from build123d import *

# Parameters (mm, degrees)
SKETCH_23_R                      = 1.6
SKETCH_23_R_2                    = 2.15
EXTRUDE_9_DEPTH                  = 12
SKETCH_25_R                      = 3.199536645
SKETCH_25_R_2                    = 3.253572192
SKETCH_25_R_3                    = 3.504037636
EXTRUDE_11_DEPTH                 = 8.5
SKETCH_27_R                      = 2.9
CUT_EXTRUDE_14_DEPTH             = 15
CUT_EXTRUDE_14_DEPTH_BACK        = 5
EXTRUDE_14_DEPTH                 = 48
EXTRUDE_14_DEPTH_BACK            = 8.5
EXTRUDE_15_REACH                 = 62
SKETCH_30_R                      = 2.823102459
SKETCH_30_R_2                    = 3.099807243
CUT_EXTRUDE_15_DEPTH             = 38
CUT_EXTRUDE_16_REACH             = 8
SKETCH_33_R                      = 1.4
CUT_EXTRUDE_16_DIRECTION_2_REACH = 56


with BuildPart() as part:
    # 草图23 → 凸台-拉伸9 (new body)
    with BuildSketch(Plane(origin=(10, 0, 0), x_dir=(0, 0, -1), z_dir=(1, 0, 0))):
        with BuildLine():
            Line((32.5, 0), (32.5, 29))
            Line((32.5, 29), (27, 29))
            Line((27, 29), (27, 13.076696831))
            ThreePointArc((27, 13.076696831), (-30, 0), (27, -13.076696831))
            Line((27, -13.076696831), (27, -29))
            Line((27, -29), (32.5, -29))
            Line((32.5, -29), (32.5, 0))
        make_face()
        with Locations((0, 12.5)):
            Circle(SKETCH_23_R, mode=Mode.SUBTRACT)
        with Locations((-10.825317547, 6.25)):
            Circle(SKETCH_23_R, mode=Mode.SUBTRACT)
        with Locations((10.825317547, 6.25)):
            Circle(SKETCH_23_R, mode=Mode.SUBTRACT)
        with Locations((10.825317547, -6.25)):
            Circle(SKETCH_23_R, mode=Mode.SUBTRACT)
        with Locations((0, -12.5)):
            Circle(SKETCH_23_R, mode=Mode.SUBTRACT)
        with Locations((-10.825317547, -6.25)):
            Circle(SKETCH_23_R, mode=Mode.SUBTRACT)
        with Locations((5.1, 8.833459119)):
            Circle(SKETCH_23_R_2, mode=Mode.SUBTRACT)
        with Locations((-10.2, 0)):
            Circle(SKETCH_23_R_2, mode=Mode.SUBTRACT)
        with Locations((5.1, -8.833459119)):
            Circle(SKETCH_23_R_2, mode=Mode.SUBTRACT)
    extrude(amount=-EXTRUDE_9_DEPTH)

    # 草图25 → 凸台-拉伸11 (add)
    with BuildSketch(Plane(origin=(10, 0, 0), x_dir=(0, 0, -1), z_dir=(1, 0, 0))):
        with Locations((5.1, 8.833459119)):
            Circle(SKETCH_25_R)
        with Locations((-10.2, 0)):
            Circle(SKETCH_25_R_2)
        with Locations((5.1, -8.833459119)):
            Circle(SKETCH_25_R_3)
    extrude(amount=-EXTRUDE_11_DEPTH)

    # 草图27 → 切除-拉伸14 (cut, two sides)
    with BuildSketch(Plane(origin=(10, 0, 0), x_dir=(0, 0, -1), z_dir=(1, 0, 0))) as cut_extrude_14_sk:
        with Locations((0, 12.5)):
            Circle(SKETCH_27_R)
        with Locations((-86.65969357, 123.729949726)):
            Circle(SKETCH_27_R)
        with Locations((-33.661578231, 254.394420705)):
            Circle(SKETCH_27_R)
        with Locations((105.996230679, 273.828941958)):
            Circle(SKETCH_27_R)
        with Locations((192.655924249, 162.598992232)):
            Circle(SKETCH_27_R)
        with Locations((139.657808909, 31.934521253)):
            Circle(SKETCH_27_R)
        with Locations((10.825317547, 6.25)):
            Circle(SKETCH_27_R)
        with Locations((10.825317547, -6.25)):
            Circle(SKETCH_27_R)
        with Locations((0, -12.5)):
            Circle(SKETCH_27_R)
        with Locations((-10.825317547, -6.25)):
            Circle(SKETCH_27_R)
        with Locations((-10.825317547, 6.25)):
            Circle(SKETCH_27_R)
    extrude(amount=CUT_EXTRUDE_14_DEPTH, mode=Mode.SUBTRACT)
    extrude(cut_extrude_14_sk.sketch, amount=-CUT_EXTRUDE_14_DEPTH_BACK, mode=Mode.SUBTRACT)

    # 草图29 → 凸台-拉伸14 (add, two sides)
    with BuildSketch(Plane(origin=(10, 0, 0), x_dir=(0, 0, -1), z_dir=(1, 0, 0))) as extrude_14_sk:
        with BuildLine():
            Line((-7, 29.171904292), (-7, -29.171904292))
            ThreePointArc((-7, -29.171904292), (0, -30), (7, -29.171904292))
            Line((7, -29.171904292), (7, 29.171904292))
            ThreePointArc((7, 29.171904292), (0, 30), (-7, 29.171904292))
        make_face()
    extrude(amount=EXTRUDE_14_DEPTH)
    extrude(extrude_14_sk.sketch, amount=-EXTRUDE_14_DEPTH_BACK)

    # 草图30 → 凸台-拉伸15 (add, up to next)
    with BuildSketch(Plane.ZY.offset(2), mode=Mode.PRIVATE) as extrude_15_sk1:
        with Locations((0, 12.5)):
            Circle(SKETCH_30_R)
    extrude_15_tool1 = extrude(extrude_15_sk1.sketch, amount=-EXTRUDE_15_REACH, mode=Mode.PRIVATE) - part.part
    add(extrude_15_tool1.solids().sort_by_distance((-2, 12.5, 0))[0])
    # 草图30 → 凸台-拉伸15 (add, up to next)
    with BuildSketch(Plane.ZY.offset(2), mode=Mode.PRIVATE) as extrude_15_sk2:
        with Locations((0, -12.5)):
            Circle(SKETCH_30_R_2)
    extrude_15_tool2 = extrude(extrude_15_sk2.sketch, amount=-EXTRUDE_15_REACH, mode=Mode.PRIVATE) - part.part
    add(extrude_15_tool2.solids().sort_by_distance((-2, -12.5, 0))[0])

    # 草图32 → 切除-拉伸15 (cut, through all)
    with BuildSketch(Plane(origin=(0, 0, -7), x_dir=(-1, 0, 0), z_dir=(0, 0, -1))):
        Polygon((-58, 0), (-58, 24), (-10, 24), (-10, -24), (-58, -24), align=None)
    extrude(amount=-CUT_EXTRUDE_15_DEPTH, mode=Mode.SUBTRACT)

    # 草图33 → 切除-拉伸16 (cut, up to next)
    with BuildSketch(Plane(origin=(0, -24, 0), x_dir=(1, 0, 0), z_dir=(0, 1, 0)), mode=Mode.PRIVATE) as cut_extrude_16_sk1:
        with Locations((34.5, 0)):
            Circle(SKETCH_33_R)
    cut_extrude_16_tool1 = extrude(cut_extrude_16_sk1.sketch, amount=-CUT_EXTRUDE_16_REACH, mode=Mode.PRIVATE) & part.part
    add(cut_extrude_16_tool1.solids().sort_by_distance((34.5, -24, 0))[0], mode=Mode.SUBTRACT)
    # 草图33 → 切除-拉伸16 (cut, up to next)
    with BuildSketch(Plane(origin=(0, -24, 0), x_dir=(1, 0, 0), z_dir=(0, 1, 0)), mode=Mode.PRIVATE) as cut_extrude_16_sk2:
        with Locations((42, 0)):
            Circle(SKETCH_33_R)
    cut_extrude_16_tool2 = extrude(cut_extrude_16_sk2.sketch, amount=-CUT_EXTRUDE_16_REACH, mode=Mode.PRIVATE) & part.part
    add(cut_extrude_16_tool2.solids().sort_by_distance((42, -24, 0))[0], mode=Mode.SUBTRACT)
    # 草图33 → 切除-拉伸16 (cut, up to next)
    with BuildSketch(Plane(origin=(0, -24, 0), x_dir=(1, 0, 0), z_dir=(0, 1, 0)), mode=Mode.PRIVATE) as cut_extrude_16_sk3:
        with Locations((27, 0)):
            Circle(SKETCH_33_R)
    cut_extrude_16_tool3 = extrude(cut_extrude_16_sk3.sketch, amount=-CUT_EXTRUDE_16_REACH, mode=Mode.PRIVATE) & part.part
    add(cut_extrude_16_tool3.solids().sort_by_distance((27, -24, 0))[0], mode=Mode.SUBTRACT)

    # 草图33 → 切除-拉伸16 direction 2 (cut, up to next)
    with BuildSketch(Plane(origin=(0, -24, 0), x_dir=(1, 0, 0), z_dir=(0, 1, 0)), mode=Mode.PRIVATE) as cut_extrude_16_direction_2_sk1:
        with Locations((34.5, 0)):
            Circle(SKETCH_33_R)
    cut_extrude_16_direction_2_tool1 = extrude(cut_extrude_16_direction_2_sk1.sketch, amount=CUT_EXTRUDE_16_DIRECTION_2_REACH, mode=Mode.PRIVATE) & part.part
    add(cut_extrude_16_direction_2_tool1.solids().sort_by_distance((34.5, -24, 0))[0], mode=Mode.SUBTRACT)
    # 草图33 → 切除-拉伸16 direction 2 (cut, up to next)
    with BuildSketch(Plane(origin=(0, -24, 0), x_dir=(1, 0, 0), z_dir=(0, 1, 0)), mode=Mode.PRIVATE) as cut_extrude_16_direction_2_sk2:
        with Locations((42, 0)):
            Circle(SKETCH_33_R)
    cut_extrude_16_direction_2_tool2 = extrude(cut_extrude_16_direction_2_sk2.sketch, amount=CUT_EXTRUDE_16_DIRECTION_2_REACH, mode=Mode.PRIVATE) & part.part
    add(cut_extrude_16_direction_2_tool2.solids().sort_by_distance((42, -24, 0))[0], mode=Mode.SUBTRACT)
    # 草图33 → 切除-拉伸16 direction 2 (cut, up to next)
    with BuildSketch(Plane(origin=(0, -24, 0), x_dir=(1, 0, 0), z_dir=(0, 1, 0)), mode=Mode.PRIVATE) as cut_extrude_16_direction_2_sk3:
        with Locations((27, 0)):
            Circle(SKETCH_33_R)
    cut_extrude_16_direction_2_tool3 = extrude(cut_extrude_16_direction_2_sk3.sketch, amount=CUT_EXTRUDE_16_DIRECTION_2_REACH, mode=Mode.PRIVATE) & part.part
    add(cut_extrude_16_direction_2_tool3.solids().sort_by_distance((27, -24, 0))[0], mode=Mode.SUBTRACT)


solid = part.part
The listing builds one solid part. Answer for the finished solid, in the listing's coordinates (mm). A direction names the side the tool comes from. Round coordinates to 2 decimals unless told otherwise and drop trailing zeros. Write each loop counter-clockwise with the first axis right and the second up, starting at its lowest first coordinate (ties: lowest second). Pieces come first, ordered by that corner, then holes. Notation, with made-up numbers: (-7, 60.25) - (23, 60.25) arc R21 cw to (23, 75.25) - close; hole circle Ø2 at (67.5, -2.5). An arc over 180 degrees is marked (long way). Use one line per item in the form item = value. Start each with the question number.
Item 1: Determine the mould class of faces 1 (the cylindrical face through (33.1, -26.96, -0.06)), 2 (the flat face through (4, -29, -30)), 3 (the flat face through (1.5, 0, 10)) for opening direction Y: +Y half, -Y half, draft (parallel to the pull), parting line (faces both ways), or undercut.
Item 2: A cutting plane is placed at C-C (y = -17). Write down the section's boundary in (x, z).
Item 3: A cutting plane is placed at D-D (y = 0). Write down the section's boundary in (x, z).
Item 4: A cutting plane is placed at A-A (z = 0). Give the number of separate pieces and of enclosed holes in the cut face, plus the area to 3 significant figures.
Item 5: A cutting plane is placed at B-B (x = 47.5). Write down the section's boundary in (y, z).
Item 6: Find the intervals of material crossed by line 1 (X direction, y = -28, z = 0); line 2 (Z direction, x = 42, y = -28); line 3 (Y direction, x = -0.3, z = -5.1), in increasing order. Write a range as [from, to].
Item 7: A tool of negligible diameter and unlimited length cuts with its end or side. For faces 4 (the flat face through (34, 27, 7)), 5 (the flat face through (5, 5, -12.1)), 6 (the flat face through (34, -27, -7)), 7 (the flat face through (34, -24, -2)), from which of +Z, -Z, +X, -X, +Y, -Y can it reach the whole face along a straight path? Write none if from no direction.
Item 8: Flat-ended cylindrical pins translate along their axes: pin 1 Ø2 at (y, z) = (-9.5, -5) entering from -X; pin 2 Ø3.5 at (x, y) = (1, 23.5) entering from +Z; pin 3 Ø4 at (x, y) = (29.5, 26) entering from -Z; pin 4 Ø4.5 at (y, z) = (0, 10) entering from -X. Find the tip coordinate at first contact, or state that the pin passes through.
The answers:
q1.face_1 = draft
q1.face_2 = -Y half
q1.face_3 = undercut
q2.outline = (-2, -32.5) - (10, -32.5) - (10, -27) - (-2, -27) - close; (-2, -24.72) - (10, -24.72) - (10, 24.72) - (-2, 24.72) - close
q3.outline = (-2, -32.5) - (10, -32.5) - (10, 30) - (-2, 30) - (-2, 12.35) - (1.5, 12.35) - (1.5, 8.05) - (-2, 8.05) - close
q4.separate_pieces = 7
q4.enclosed_holes = 0
q4.area = 1,200 mm^2
q5.outline = (-29.17, -7) - (-24, -7) - (-24, 7) - (-29.17, 7) arc R30 ccw to start; (24, -7) - (29.17, -7) arc R30 ccw to (29.17, 7) - (24, 7) - close
q6.line_1 = [-2, 25.6], [28.4, 33.1], [35.9, 40.6], [43.4, 58]
q6.line_2 = [-7, -1.4], [1.4, 7]
q6.line_3 = [-29.56, -10.98], [-6.68, 6.68], [10.98, 29.56]
q7.face_4 = +Z, +X, +Y, -Y
q7.face_5 = +X
q7.face_6 = -Z, +X, +Y, -Y
q7.face_7 = +Z, -Z, +X
q8.pin_1 = 1.5
q8.pin_2 = 20.66
q8.pin_3 = -7
q8.pin_4 = -2
